from build123d import *

# Parameters (mm, degrees)
F0_R     = 9.525
F1_DEPTH = 6.35


with BuildPart() as f1:
    # F0 (on Top) → F1 (new body)
    with BuildSketch(Plane.XY):
        with BuildLine():
            Line((34.570389, 57.15), (-54.329611, 57.15))
            ThreePointArc((-54.329611, 57.15), (-67.799996, 51.570384), (-73.379611, 38.1))
            Line((-73.379611, 38.1), (-73.379611, 15.24))
            Line((-73.379611, 15.24), (-31.425689, 15.24))
            ThreePointArc((-31.425689, 15.24), (-14.821988, 26.515286), (4.852767, 30.48))
            ThreePointArc((4.852767, 30.48), (12.036972, 27.504205), (15.012767, 20.32))
            Line((15.012767, 20.32), (64.796767, 20.32))
            Line((64.796767, 20.32), (64.796767, 0))
            Line((64.796767, 0), (64.796767, -20.32))
            Line((64.796767, -20.32), (15.012767, -20.32))
            ThreePointArc((15.012767, -20.32), (12.036972, -27.504205), (4.852767, -30.48))
            ThreePointArc((4.852767, -30.48), (-14.821988, -26.515286), (-31.425689, -15.24))
            Line((-31.425689, -15.24), (-73.379611, -15.24))
            Line((-73.379611, -15.24), (-73.379611, -38.1))
            ThreePointArc((-73.379611, -38.1), (-67.799996, -51.570384), (-54.329611, -57.15))
            Line((-54.329611, -57.15), (34.570389, -57.15))
            Line((34.570389, -57.15), (75.210389, -46.260545))
            Line((75.210389, -46.260545), (88.672767, -32.798166))
            Line((88.672767, -32.798166), (88.672767, 0))
            Line((88.672767, 0), (88.672767, 32.798166))
            Line((88.672767, 32.798166), (75.210389, 46.260545))
            Line((75.210389, 46.260545), (34.570389, 57.15))
        make_face()
        with Locations((-54.329611, -38.1)):
            Circle(F0_R, mode=Mode.SUBTRACT)
        with Locations((34.570389, -38.1)):
            Circle(F0_R, mode=Mode.SUBTRACT)
        with Locations((-54.329611, 38.1)):
            Circle(F0_R, mode=Mode.SUBTRACT)
        with Locations((34.570389, 38.1)):
            Circle(F0_R, mode=Mode.SUBTRACT)
    extrude(amount=F1_DEPTH)


solid = f1.part
Model file for the job. Use its own axes, mm. A direction names the side the tool comes from. Give positions to 0.01 mm unless a question says otherwise; leave off trailing zeros. Loops run counter-clockwise (first coordinate to the right, second up) from the corner with the lowest first, then second, coordinate; pieces in that order, holes last.
1) Pull direction X, two halves, no side cores. Call faces 1 (the flat face through (-73.38, 27, 3)), 2 (the flat face through (40, 20.32, 3)), 3 (the flat face through (25, -25, 6.35)): +X half, -X half, draft (parallel to the pull), parting line (faces both ways), or undercut.
2) Wall check: line 1 (X direction, y = 38, z = 4.5); line 2 (Y direction, x = -58.5, z = 1.5); line 3 (X direction, y = -15, z = 2.25). Give the ranges that are in metal, low to high.
3) Saw through at D-D (x = -43). Write the cut outline in (y, z), plus the area to 3 significant figures.
4) Flat gauge pins, fed straight in: pin 1 Ø1.9 at (x, z) = (36.5, 3) entering from +Y; pin 2 Ø3 at (y, z) = (7, 2) entering from -X. Where does each tip first touch, or does it go through?
5) Saw through at C-C (x = 41.5). Write the cut outline in (y, z) (3 decimals).
6) Saw through at B-B (z = 3.75). Write the cut outline in (x, y) (3 decimals).
7) Tool access for faces 4 (the flat face through (-53, 15.24, 3)), 5 (the cylindrical face through (-15.082, 26.405, 3.131)), 6 (the flat face through (82.036, 39.435, 3.131)): list every direction of +Z, -Z, +X, -X, +Y, -Y with a clear straight run to the whole face (end or side of a thin tool).
8) Saw through at A-A (x = 22.5). Write the cut outline in (y, z).
Answer block:
1. face 1: -X half
1. face 2: undercut
1. face 3: draft
2. line 1: x = -73.38 to -63.85, -44.81 to 25.05, 44.09 to 83.47
2. line 2: y = -56.69 to -46.66, -29.54 to -15.24, 15.24 to 29.54, 46.66 to 56.69
2. line 3: x = 64.8 to 88.67
3. outline: (-57.15, 0) - (-15.24, 0) - (-15.24, 6.35) - (-57.15, 6.35) - close; (15.24, 0) - (57.15, 0) - (57.15, 6.35) - (15.24, 6.35) - close
3. area: 532 mm2
4. pin 1: stops at y = 56.89
4. pin 2: stops at x = 64.8
5. outline: (-55.293, 0) - (-44.635, 0) - (-44.635, 6.35) - (-55.293, 6.35) - close; (-31.565, 0) - (-20.32, 0) - (-20.32, 6.35) - (-31.565, 6.35) - close; (20.32, 0) - (31.565, 0) - (31.565, 6.35) - (20.32, 6.35) - close; (44.635, 0) - (55.293, 0) - (55.293, 6.35) - (44.635, 6.35) - close
6. outline: (-73.38, -38.1) arc R19.05 ccw to (-54.33, -57.15) - (34.57, -57.15) - (75.21, -46.261) - (88.673, -32.798) - (88.673, 32.798) - (75.21, 46.261) - (34.57, 57.15) - (-54.33, 57.15) arc R19.05 ccw to (-73.38, 38.1) - (-73.38, 15.24) - (-31.426, 15.24) arc R50.8 cw to (4.853, 30.48) arc R10.16 cw to (15.013, 20.32) - (64.797, 20.32) - (64.797, -20.32) - (15.013, -20.32) arc R10.16 cw to (4.853, -30.48) arc R50.8 cw to (-31.426, -15.24) - (-73.38, -15.24) - close; hole circle Ø19.05 at (-54.33, -38.1); hole circle Ø19.05 at (-54.33, 38.1); hole circle Ø19.05 at (34.57, -38.1); hole circle Ø19.05 at (34.57, 38.1)
7. face 4: +Z, -Z, -X
7. face 5: +Z, -Z
7. face 6: +Z, -Z, +X, +Y
8. outline: (-57.15, 0) - (-20.32, 0) - (-20.32, 6.35) - (-57.15, 6.35) - close; (20.32, 0) - (57.15, 0) - (57.15, 6.35) - (20.32, 6.35) - close
